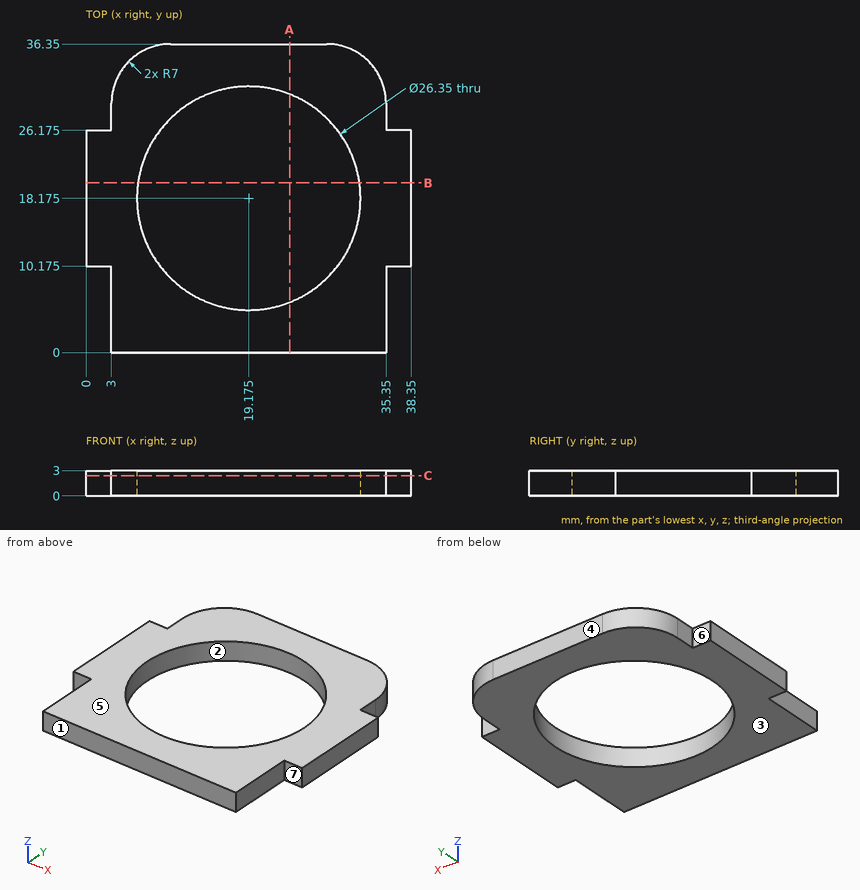
Check sheet for the drawn part. Datum: minimum x, y, z corner. Units: mm. A direction names the side the tool comes from. Give positions to 0.01 mm unless a question says otherwise; leave off trailing zeros. Order: outer loops, then holes, each group sorted by start corner. A loop starts at its lowest first (then second) coordinate and runs counter-clockwise, first axis right, second up. Notation, with made-up numbers: (-18.75, -14.5) - (19.25, -14.5) arc R24 ccw to (19.25, 1.5) - close; hole circle Ø3 at (-14.75, 56.25). An arc over 180 degrees is marked (long way). Answer as a JSON object with one key per item and string values.
(1) Cross-section at A-A (x = 24). Record the cut outline in (y, z).
Report:
{"outline": "(0, 0) - (5.92, 0) - (5.92, 3) - (0, 3) - close; (30.43, 0) - (36.35, 0) - (36.35, 3) - (30.43, 3) - close"}
(2) Tool access check on the marked faces 5, 6 and 7. Record the directions out of +Z, -Z, +X, -X, +Y, -Y that give a thin tool (end or side, any length) a straight path to the whole face; none if there is none.
Report:
{"face 5": "+Z, +X, -X, +Y, -Y", "face 6": "+Z, -Z, -X, +Y", "face 7": "+Z, -Z, +X, -Y"}
(3) Depth check by flat-ended pin: pin 1 Ø1.5 at (y, z) = (31.5, 2) entering from -X; pin 2 Ø0.9 at (x, z) = (36.5, 1) entering from -Y (3 decimals); pin 3 Ø0.9 at (y, z) = (7, 2) entering from -X. Enter the tip coordinate at first touch or a pass-through.
Report:
{"pin 1": "x = 3.14", "pin 2": "y = 10.175", "pin 3": "x = 3"}
(4) Cross-section at B-B (y = 20). Record the cut outline in (x, z).
Report:
{"outline": "(0, 0) - (6.13, 0) - (6.13, 3) - (0, 3) - close; (32.22, 0) - (38.35, 0) - (38.35, 3) - (32.22, 3) - close"}
(5) Cross-section at C-C (z = 2.4). Record the cut outline in (x, y) (3 decimals).
Report:
{"outline": "(0, 10.175) - (3, 10.175) - (3, 0) - (35.35, 0) - (35.35, 10.175) - (38.35, 10.175) - (38.35, 26.175) - (35.35, 26.175) - (35.35, 29.35) arc R7 ccw to (28.35, 36.35) - (10, 36.35) arc R7 ccw to (3, 29.35) - (3, 26.175) - (0, 26.175) - close; hole circle Ø26.35 at (19.175, 18.175)"}
(6) Material ranges on line 1 (X direction, y = 6, z = 2.85); line 2 (Y direction, x = 16, z = 0.3); line 3 (X direction, y = 10.5, z = 0.65), recorded low to high.
Report:
{"line 1": "3 to 14.14, 24.21 to 35.35", "line 2": "0 to 5.39, 30.96 to 36.35", "line 3": "0 to 8.47, 29.88 to 38.35"}
(7) Draft check along Y on the marked faces 1, 2, 3 and 4. Enter one of: released by +Y, released by -Y, zero draft, split by the parting line, or undercut.
Report:
{"face 1": "released by -Y", "face 2": "undercut", "face 3": "zero draft", "face 4": "released by +Y"}
